from build123d import *

# Parameters (mm, degrees)
SKETCH_1_W                = 130
SKETCH_1_H                = 15
EXTRUDE_1_DEPTH           = 8
CUT_EXTRUDE_10_REACH      = 133.107
SKETCH_17_R               = 3
SKETCH_19_W               = 8
SKETCH_19_H               = 15
EXTRUDE_6_DEPTH           = 117.2
FILLET_1_R                = 5
CUT_EXTRUDE_12_REACH      = 133.107
SKETCH_15_R               = 3
SKETCH_22_W               = 8
SKETCH_22_H               = 8
EXTRUDE_7_DEPTH           = 5
CUT_EXTRUDE_18_DEPTH      = 1.5
SKETCH_25_W               = 4.62
SKETCH_25_H               = 1.5
CUT_EXTRUDE_19_DEPTH      = 4
FILLET_8_R                = 3
FILLET_9_R                = 2
FILLET_10_R               = 2
FILLET_11_R               = 3
CUT_EXTRUDE_20_DEPTH      = 15.5
CUT_EXTRUDE_20_DEPTH_BACK = 28.5
SKETCH_21_R               = 1


with BuildPart() as part:
    # Sketch 1 → Extrude 1 (new body)
    with BuildSketch(Plane(origin=(0, 0, 0), x_dir=(0, 0, -1), z_dir=(1, 0, 0))):
        with Locations((65, 7.5)):
            Rectangle(SKETCH_1_W, SKETCH_1_H)
    extrude(amount=EXTRUDE_1_DEPTH)

    # Sketch 17 → Cut-Extrude 10 (cut, up to next)
    with BuildSketch(Plane.ZY, mode=Mode.PRIVATE) as cut_extrude_10_sk1:
        with Locations((-115, 7.5)):
            Circle(SKETCH_17_R)
    cut_extrude_10_tool1 = extrude(cut_extrude_10_sk1.sketch, amount=-CUT_EXTRUDE_10_REACH, mode=Mode.PRIVATE) & part.part
    # Sketch 17 → Cut-Extrude 10 (cut, up to next)
    with BuildSketch(Plane.ZY, mode=Mode.PRIVATE) as cut_extrude_10_sk2:
        with Locations((-95, 7.5)):
            Circle(SKETCH_17_R)
    cut_extrude_10_tool2 = extrude(cut_extrude_10_sk2.sketch, amount=-CUT_EXTRUDE_10_REACH, mode=Mode.PRIVATE) & part.part
    # Sketch 17 → Cut-Extrude 10 (cut, up to next)
    with BuildSketch(Plane.ZY, mode=Mode.PRIVATE) as cut_extrude_10_sk3:
        with Locations((-75, 7.5)):
            Circle(SKETCH_17_R)
    cut_extrude_10_tool3 = extrude(cut_extrude_10_sk3.sketch, amount=-CUT_EXTRUDE_10_REACH, mode=Mode.PRIVATE) & part.part
    # Sketch 17 → Cut-Extrude 10 (cut, up to next)
    with BuildSketch(Plane.ZY, mode=Mode.PRIVATE) as cut_extrude_10_sk4:
        with Locations((-55, 7.5)):
            Circle(SKETCH_17_R)
    cut_extrude_10_tool4 = extrude(cut_extrude_10_sk4.sketch, amount=-CUT_EXTRUDE_10_REACH, mode=Mode.PRIVATE) & part.part
    # Sketch 17 → Cut-Extrude 10 (cut, up to next)
    with BuildSketch(Plane.ZY, mode=Mode.PRIVATE) as cut_extrude_10_sk5:
        with Locations((-35, 7.5)):
            Circle(SKETCH_17_R)
    cut_extrude_10_tool5 = extrude(cut_extrude_10_sk5.sketch, amount=-CUT_EXTRUDE_10_REACH, mode=Mode.PRIVATE) & part.part
    cut_extrude_10_1 = cut_extrude_10_tool1.solids().sort_by_distance((0, 7.5, -115))[0]
    add(cut_extrude_10_1, mode=Mode.SUBTRACT)
    cut_extrude_10_2 = cut_extrude_10_tool2.solids().sort_by_distance((0, 7.5, -95))[0]
    add(cut_extrude_10_2, mode=Mode.SUBTRACT)
    cut_extrude_10_3 = cut_extrude_10_tool3.solids().sort_by_distance((0, 7.5, -75))[0]
    add(cut_extrude_10_3, mode=Mode.SUBTRACT)
    cut_extrude_10_4 = cut_extrude_10_tool4.solids().sort_by_distance((0, 7.5, -55))[0]
    add(cut_extrude_10_4, mode=Mode.SUBTRACT)
    cut_extrude_10_5 = cut_extrude_10_tool5.solids().sort_by_distance((0, 7.5, -35))[0]
    add(cut_extrude_10_5, mode=Mode.SUBTRACT)
    cut_extrude_10 = cut_extrude_10_1 + cut_extrude_10_2 + cut_extrude_10_3 + cut_extrude_10_4 + cut_extrude_10_5  # Cut-Extrude 10 as one shape, for the pattern or mirror that repeats it

    # Sketch 19 → Extrude 6 (add)
    with BuildSketch(Plane.XY):
        with Locations((4, 7.5)):
            Rectangle(SKETCH_19_W, SKETCH_19_H)
    extrude(amount=EXTRUDE_6_DEPTH)

    # Mirror 1: Cut-Extrude 10 across plane
    add(cut_extrude_10.mirror(Plane.XY.offset(-6.4)), mode=Mode.SUBTRACT)

    # Fillet 1
    fillet_1_edges = [part.edges().sort_by_distance(p)[0] for p in [
        (4, 0, 117.2),
        (4, 15, 117.2),
        (4, 15, -130),
        (4, 0, -130),
    ]]
    fillet(fillet_1_edges, radius=FILLET_1_R)

    # Sketch 15 → Cut-Extrude 12 (cut, up to next)
    with BuildSketch(Plane.ZY, mode=Mode.PRIVATE) as cut_extrude_12_sk1:
        with Locations((-6.4, 7.5)):
            Circle(SKETCH_15_R)
    cut_extrude_12_tool1 = extrude(cut_extrude_12_sk1.sketch, amount=-CUT_EXTRUDE_12_REACH, mode=Mode.PRIVATE) & part.part
    add(cut_extrude_12_tool1.solids().sort_by_distance((0, 7.5, -6.4))[0], mode=Mode.SUBTRACT)

    # Sketch 22 → Extrude 7 (add)
    with BuildSketch(Plane(origin=(0, 15, 0), x_dir=(1, 0, 0), z_dir=(0, 1, 0))):
        with Locations((4, 6.4)):
            Rectangle(SKETCH_22_W, SKETCH_22_H)
    extrude_7 = extrude(amount=EXTRUDE_7_DEPTH)

    # Sketch 24 → Cut-Extrude 18 (cut)
    with BuildSketch(Plane(origin=(0, 15, 0), x_dir=(1, 0, 0), z_dir=(0, 1, 0))):
        Polygon((4, 4.090598923), (6, 5.245299462), (6, 7.554700538), (4, 8.709401077), (2, 7.554700538), (2, 5.245299462), align=None)
    cut_extrude_18 = extrude(amount=CUT_EXTRUDE_18_DEPTH, mode=Mode.SUBTRACT)

    # Sketch 25 → Cut-Extrude 19 (cut)
    with BuildSketch(Plane(origin=(8, 0, 0), x_dir=(0, 0, -1), z_dir=(1, 0, 0))):
        with Locations((6.4, 15.75)):
            Rectangle(SKETCH_25_W, SKETCH_25_H)
    cut_extrude_19 = extrude(amount=-CUT_EXTRUDE_19_DEPTH, mode=Mode.SUBTRACT)

    # Fillet 8
    fillet_8_edges = [part.edges().sort_by_distance(p)[0] for p in [
        (4, 15, -2.4),
        (4, 15, -10.4),
    ]]
    fillet(fillet_8_edges, radius=FILLET_8_R)

    # Fillet 9
    fillet_9_edges = [part.edges().sort_by_distance(p)[0] for p in [
        (4, 20, -2.4),
        (4, 20, -10.4),
    ]]
    fillet(fillet_9_edges, radius=FILLET_9_R - 0.0001)  # a hair under: the kernel refuses the full size

    # Mirror 6: Extrude 7, Cut-Extrude 18, Cut-Extrude 19 across plane
    add(extrude_7.mirror(Plane.ZX.offset(7.5)))
    add(cut_extrude_18.mirror(Plane.ZX.offset(7.5)), mode=Mode.SUBTRACT)
    add(cut_extrude_19.mirror(Plane.ZX.offset(7.5)), mode=Mode.SUBTRACT)

    # Fillet 10
    fillet_10_edges = [part.edges().sort_by_distance(p)[0] for p in [
        (4, -5, -10.4),
        (4, -5, -2.4),
    ]]
    fillet(fillet_10_edges, radius=FILLET_10_R)

    # Fillet 11
    fillet_11_edges = [part.edges().sort_by_distance(p)[0] for p in [
        (4, 0, -2.4),
        (4, 0, -10.4),
    ]]
    fillet(fillet_11_edges, radius=FILLET_11_R - 0.0001)  # a hair under: the kernel refuses the full size

    # Sketch 21 → Cut-Extrude 20 (cut, two sides: drawn at the far end of the back side and taken through both)
    with BuildSketch(Plane(origin=(0, 15, 0), x_dir=(1, 0, 0), z_dir=(0, 1, 0)).offset(-CUT_EXTRUDE_20_DEPTH_BACK)):
        with Locations(Location((4, 6.4, 0), (0, 0, 90))):
            Circle(SKETCH_21_R)
    extrude(amount=CUT_EXTRUDE_20_DEPTH + CUT_EXTRUDE_20_DEPTH_BACK, mode=Mode.SUBTRACT)


solid = part.part
For this review, take the finished solid that the model builds, in its own axes (mm). A direction names the side the tool comes from. Give positions to 0.01 mm unless a question says otherwise; leave off trailing zeros. Loops run counter-clockwise (first coordinate to the right, second up) from the corner with the lowest first, then second, coordinate; pieces in that order, holes last. Notation, with made-up numbers: M 25,-3.5 L 35,-3.5 A24 cw 35,29.5 Z; hole C -6,-17 d9. An arc over 180 degrees is marked long. Put each result on its own line as item: value. Start each with the question number.
(1) Add section A-A, the plane z = -75. Write out the cut boundary in (x, y).
(2) For pin 1 (2 mm diameter, centred on x = 6, z = 28.5, fed in from +Y); pin 2 (1.2 mm diameter, centred on y = -0.5, z = -6, fed in from +X); pin 3 (5.5 mm diameter, centred on y = 7.5, z = -75, fed in from -X); pin 4 (1 mm diameter, centred on x = 4, y = 13, fed in from -Z), all flat-tipped, find the tip position at first contact; note any pin that passes through.
(3) Wall thickness on L1, parallel to Y at x = 7.75, z = -75.5; L2, parallel to Y at x = 4.25, z = -88; L3, parallel to Y at x = 2.5, z = -56.5: over which ranges is each line inside the solid? List them lowest first.
(4) Machinability: for faces 1 (the flat face through (6, 15, -6)), 2 (the flat face through (4, 15, 56)), 3 (the cylindrical face through (3.94, 8.4, 59.34)), which of the approach directions +Z, -Z, +X, -X, +Y, -Y give a long, thin tool a straight path to every point of the face, cutting with its end or side? Answer none if there is none.
(5) Add section B-B, the plane z = 94.5. Write out the cut boundary in (x, y), then the cut area to 3 significant figures.
(6) The part is to be moulded in two halves that separate along Z. For faces 4 (the flat face through (4, 7, -130)), 5 (the flat face through (4, 0, 56)), 6 (the cylindrical face through (3.944, 4.838, -5.016)), say which applies: +Z half, -Z half, draft (parallel to the pull), parting line (faces both ways), or undercut.
Result:
1. outline: M 0,0 L 8,0 L 8,4.5 L 0,4.5 Z; M 0,10.5 L 8,10.5 L 8,15 L 0,15 Z
2. pin 1: stops at y = 15
2. pin 2: stops at x = 8
2. pin 3: passes through
2. pin 4: stops at z = -129.33
3. L1: y = 0 to 4.54, 10.46 to 15
3. L2: y = 0 to 15
3. L3: y = 0 to 4.9, 10.1 to 15
4. face 1: +X
4. face 2: +Z, +X, -X, +Y
4. face 3: +X, -X
5. outline: M 0,0 L 8,0 L 8,15 L 0,15 Z
5. area: 120 mm^2
6. face 4: -Z half
6. face 5: draft
6. face 6: undercut
